Geometry check sheet. Reference: drawing and pictorial views, mm from the part's lowest x, y, z. Round coordinates to 2 decimals unless told otherwise and drop trailing zeros. Loops run counter-clockwise (first coordinate to the right, second up) from the corner with the lowest first, then second, coordinate; pieces in that order, holes last. Notation, with made-up numbers: (9.5, -16) - (13.5, -16) arc R22 ccw to (13.5, -9) - close; hole circle Ø1 at (69, 73). An arc over 180 degrees is marked (long way). Put each result on its own line as item: value. Start each with the question number.
Item 1: Section check C-C, the plane z = 29. Record the cut outline in (x, y).
Item 2: Section check B-B, the plane z = 40. Record the cut outline in (x, y), and give its area (3 significant figures).
Item 3: Gauge pin test, flat ends, axial feed: pin 1 Ø2 at (x, y) = (36, 2.5) entering from +Z; pin 2 Ø2 at (y, z) = (2, 46.5) entering from -X. Record the tip position at first contact, or that the pin passes through.
Item 4: Material ranges on line 1 along X through (y, z) = (1.25, 5); line 2 along X through (y, z) = (0.6, 28.5); line 3 along Z through (x, y) = (75, 1.6), recorded low to high.
Item 5: Section check D-D, the plane y = 3.5. Give the number of separate pieces and of enclosed holes in the cut face, and give its area (3 significant figures).
Item 6: Section check A-A, the plane x = 75. Record the cut outline in (y, z).
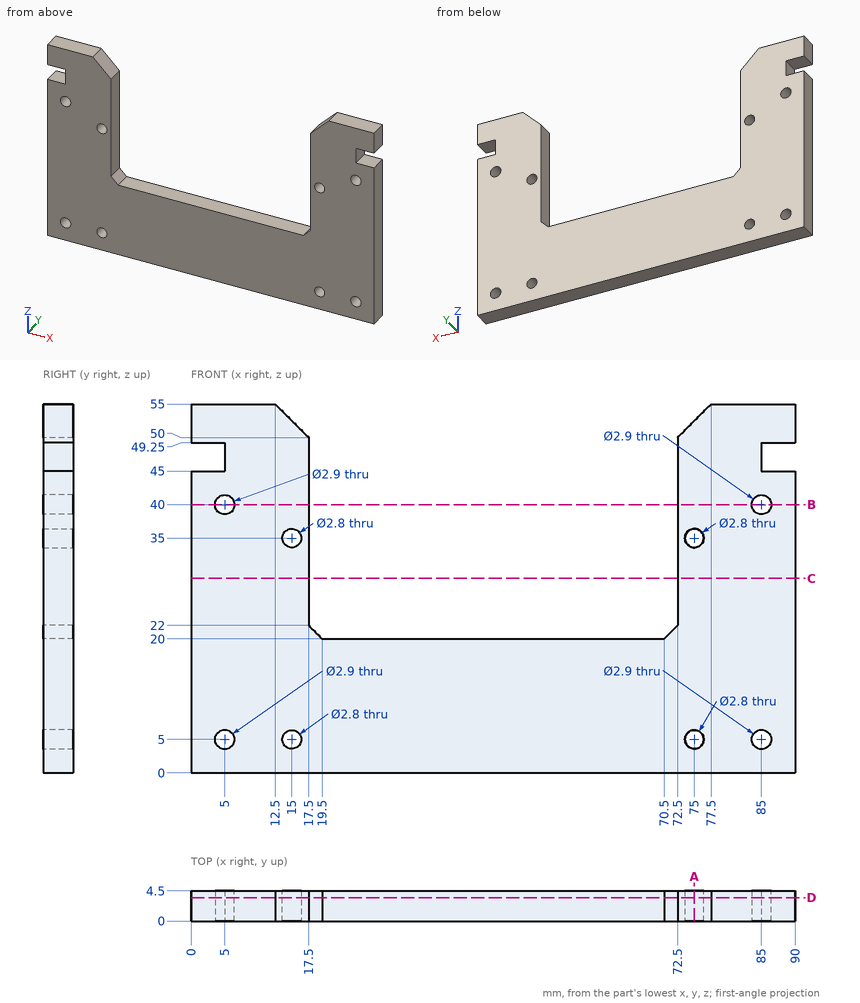
Check result:
1. outline: (0, 0) - (17.5, 0) - (17.5, 4.5) - (0, 4.5) - close; (72.5, 0) - (90, 0) - (90, 4.5) - (72.5, 4.5) - close
2. outline: (0, 0) - (3.55, 0) - (3.55, 4.5) - (0, 4.5) - close; (6.45, 0) - (17.5, 0) - (17.5, 4.5) - (6.45, 4.5) - close; (72.5, 0) - (83.55, 0) - (83.55, 4.5) - (72.5, 4.5) - close; (86.45, 0) - (90, 0) - (90, 4.5) - (86.45, 4.5) - close
2. area: 131 mm²
3. pin 1: z = 20
3. pin 2: x = 5
4. line 1: 0 to 3.55, 6.45 to 13.6, 16.4 to 73.6, 76.4 to 83.55, 86.45 to 90
4. line 2: 0 to 17.5, 72.5 to 90
4. line 3: 0 to 3.6, 6.4 to 33.6, 36.4 to 52.5
5. separate pieces: 1
5. enclosed holes: 8
5. area: 2,910 mm²
6. outline: (0, 0) - (4.5, 0) - (4.5, 3.6) - (0, 3.6) - close; (0, 6.4) - (4.5, 6.4) - (4.5, 33.6) - (0, 33.6) - close; (0, 36.4) - (4.5, 36.4) - (4.5, 52.5) - (0, 52.5) - close
